from build123d import *

# Parameters (mm, degrees)
SKETCH1_W           = 304.8
SKETCH1_H           = 190.5
BOSS_EXTRUDE1_DEPTH = 2.778125
SKETCH2_W           = 304.8
SKETCH2_H           = 19.05
CUT_EXTRUDE1_DEPTH  = 3.778125
CUT_EXTRUDE2_DEPTH  = 3.778125
SKETCH4_R           = 1.7526
CUT_EXTRUDE3_DEPTH  = 3.778125
SKETCH5_W           = 9.525
SKETCH5_H           = 171.45
CUT_EXTRUDE4_DEPTH  = 3.778125
FILLET1_R           = 2.54


with BuildPart() as part:
    # Sketch1 → Boss-Extrude1 (new body)
    with BuildSketch(Plane(origin=(0, 0, 0), x_dir=(1, 0, 0), z_dir=(0, 1, 0))):
        with Locations((152.4, 95.25)):
            Rectangle(SKETCH1_W, SKETCH1_H)
    extrude(amount=BOSS_EXTRUDE1_DEPTH)

    # Sketch2 → Cut-Extrude1 (cut, through all)
    with BuildSketch(Plane(origin=(0, 2.778125, 0), x_dir=(1, 0, 0), z_dir=(0, 1, 0))):
        with Locations((152.4, 9.525)):
            Rectangle(SKETCH2_W, SKETCH2_H)
    extrude(amount=-CUT_EXTRUDE1_DEPTH, mode=Mode.SUBTRACT)

    # Sketch3 → Cut-Extrude2 (cut, through all)
    with BuildSketch(Plane(origin=(0, 2.778125, 0), x_dir=(1, 0, 0), z_dir=(0, 1, 0))):
        Polygon((0, 19.05), (0, 69.85), (9.525, 69.85), (9.525, 28.575), (50.8, 28.575), (50.8, 19.05), align=None)
    extrude(amount=-CUT_EXTRUDE2_DEPTH, mode=Mode.SUBTRACT)

    # Sketch4 → Cut-Extrude3 (cut, through all)
    with BuildSketch(Plane(origin=(0, 2.778125, 0), x_dir=(1, 0, 0), z_dir=(0, 1, 0))):
        with Locations((12.7, 165.1)):
            Circle(SKETCH4_R)
        with Locations((12.7, 88.9)):
            Circle(SKETCH4_R)
    extrude(amount=-CUT_EXTRUDE3_DEPTH, mode=Mode.SUBTRACT)

    # Sketch5 → Cut-Extrude4 (cut, through all)
    with BuildSketch(Plane(origin=(0, 2.778125, 0), x_dir=(1, 0, 0), z_dir=(0, 1, 0))):
        with Locations((300.0375, 104.775)):
            Rectangle(SKETCH5_W, SKETCH5_H)
    extrude(amount=-CUT_EXTRUDE4_DEPTH, mode=Mode.SUBTRACT)

    # Fillet1
    fillet1_edges = [part.edges().sort_by_distance(p)[0] for p in [
        (50.8, 1.3890625, -19.05),
        (0, 1.3890625, -69.85),
        (9.525, 1.3890625, -69.85),
        (9.525, 1.3890625, -28.575),
        (50.8, 1.3890625, -28.575),
        (295.275, 1.3890625, -19.05),
    ]]
    fillet(fillet1_edges, radius=FILLET1_R)


solid = part.part
Verification items for the finished model (mm, model axes). Give positions to 0.01 mm unless a question says otherwise; leave off trailing zeros. Loops run counter-clockwise (first coordinate to the right, second up) from the corner with the lowest first, then second, coordinate; pieces in that order, holes last.
1) Sectioned sample at A-A, the plane y = 1.9. Enter the section's corners in (x, z) (3 decimals), then the cut area to 3 significant figures.
2) Thickness scan on line 1 along Z through (x, y) = (13, 0.95) (3 decimals); line 2 along Z through (x, y) = (12.7, 1.25) (3 decimals); line 3 along X through (y, z) = (1.8, -88.9) (3 decimals). Record the ranges inside material, lowest first.
3) Sectioned sample at B-B, the plane x = 43. Enter the section's corners in (y, z) (3 decimals), then the cut area to 3 significant figures.
4) Depth check by flat-ended pin: pin 1 Ø0.8 at (x, y) = (4.5, 2) entering from +Z; pin 2 Ø0.8 at (y, z) = (1.5, -55) entering from -X (3 decimals); pin 3 Ø1.4 at (x, y) = (30.5, 1.5) entering from +Z (3 decimals). Enter the tip coordinate at first touch or a pass-through.
Answers:
1. outline: (0, -190.5) - (295.275, -190.5) - (295.275, -21.59) arc R2.54 ccw to (292.735, -19.05) - (53.34, -19.05) arc R2.54 ccw to (50.8, -21.59) - (50.8, -26.035) arc R2.54 cw to (48.26, -28.575) - (12.065, -28.575) arc R2.54 ccw to (9.525, -31.115) - (9.525, -67.31) arc R2.54 cw to (6.985, -69.85) - (2.54, -69.85) arc R2.54 ccw to (0, -72.39) - close; hole circle Ø3.505 at (12.7, -165.1); hole circle Ø3.505 at (12.7, -88.9)
1. area: 49,700 mm2
2. line 1: z = -190.5 to -166.827, -163.373 to -90.627, -87.173 to -28.575
2. line 2: z = -190.5 to -166.853, -163.347 to -90.653, -87.147 to -28.575
2. line 3: x = 0 to 10.947, 14.453 to 295.275
3. outline: (0, -190.5) - (2.778, -190.5) - (2.778, -28.575) - (0, -28.575) - close
3. area: 450 mm2
4. pin 1: stops at z = -69.85
4. pin 2: stops at x = 9.525
4. pin 3: stops at z = -28.575
